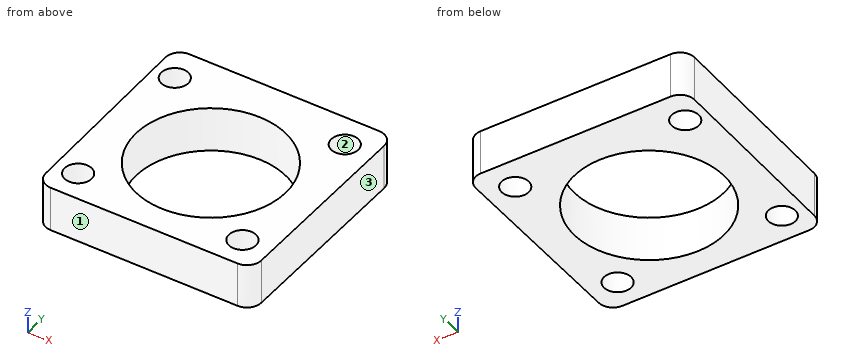
```python
from build123d import *

# Parameters (mm, degrees)
F0_R     = 7.5
F0_R_2   = 41.5
F1_DEPTH = 25


with BuildPart() as f1:
    # F0 (on Top) → F1 (new body)
    with BuildSketch(Plane.XY):
        with BuildLine():
            ThreePointArc((-59.925168, -48.84305), (-57.53589, -54.413699), (-51.926274, -56.709997))
            Line((-51.926274, -56.709997), (52.20569, -56.709997))
            ThreePointArc((52.20569, -56.709997), (57.862545, -54.366851), (60.20569, -48.709997))
            Line((60.20569, -48.709997), (60.20569, 55.273405))
            ThreePointArc((60.20569, 55.273405), (57.862545, 60.93026), (52.20569, 63.273405))
            Line((52.20569, 63.273405), (-53.655924, 63.273405))
            ThreePointArc((-53.655924, 63.273405), (-59.359626, 60.883021), (-61.654818, 55.140352))
            Line((-61.654818, 55.140352), (-59.925168, -48.84305))
        make_face()
        with Locations((-47.246009, -40.616337)):
            Circle(F0_R, mode=Mode.SUBTRACT)
        with Locations((44.347703, -40.616337)):
            Circle(F0_R, mode=Mode.SUBTRACT)
        Circle(F0_R_2, mode=Mode.SUBTRACT)
        with Locations((-49.459223, 44.541564)):
            Circle(F0_R, mode=Mode.SUBTRACT)
        with Locations((44.347703, 45.987621)):
            Circle(F0_R, mode=Mode.SUBTRACT)
    extrude(amount=-F1_DEPTH)


solid = f1.part
```
CAD build for the part. Positions are in the model's coordinates, mm. Face numbers are marked on the shaded views. Coordinates: 2 decimals unless noted, no trailing zeros. Order: outer loops, then holes, each group sorted by start corner. A loop starts at its lowest first (then second) coordinate and runs counter-clockwise, first axis right, second up. Notation, with made-up numbers: (69, 23) -> (113, 23) arc R8 ccw to (113, 34) -> close; hole circle Ø10 at (53, 8.5). An arc over 180 degrees is marked (long way). Use one line per item in the form item = value. Start each with the question number.
1) Band-saw the part on B-B on y = 0. Give the cut face in (x, z).
2) Band-saw the part on A-A on x = 0. Give the cut face in (y, z).
3) Drill centre lines: L1, parallel to Y at x = 0, z = -15.5; L2, parallel to Y at x = 46, z = -6; L3, parallel to X at y = 44, z = -12.25. Where is each one in solid material? Low to high. Write a range as [from, to].
4) Drop flat-ended pins along their axis: pin 1 (1.5 mm diameter, centred on y = 37, z = -7, fed in from -X); pin 2 (5 mm diameter, centred on y = -8.5, z = -15.5, fed in from -X); pin 3 (1 mm diameter, centred on y = 9.5, z = -8.5, fed in from -X). Give the stop position or say it passes through.
5) Pull direction X, two halves, no side cores. Call the marked faces 1, 2 and 3: +X half, -X half, draft (parallel to the pull), parting line (faces both ways), or undercut.
6) Band-saw the part on C-C on y = -43. Give the cut face in (x, z), then the cut area to 3 significant figures.
7) Band-saw the part on D-D on x = -48. Give the cut face in (y, z), then the cut area to 3 significant figures.
Entries:
q1.outline = (-60.74, -25) -> (-41.5, -25) -> (-41.5, 0) -> (-60.74, 0) -> close; (41.5, -25) -> (60.21, -25) -> (60.21, 0) -> (41.5, 0) -> close
q2.outline = (-56.71, -25) -> (-41.5, -25) -> (-41.5, 0) -> (-56.71, 0) -> close; (41.5, -25) -> (63.27, -25) -> (63.27, 0) -> (41.5, 0) -> close
q3.L1 = [-56.71, -41.5], [41.5, 63.27]
q3.L2 = [-56.71, -47.93], [-33.3, 38.67], [53.3, 63.27]
q3.L3 = [-61.47, -56.94], [-41.98, 37.12], [51.58, 60.21]
q4.pin_1 = -61.37
q4.pin_2 = -60.64
q4.pin_3 = -60.9
q5.face_1 = draft
q5.face_2 = undercut
q5.face_3 = +X half
q6.outline = (-60.02, -25) -> (-54.36, -25) -> (-54.36, 0) -> (-60.02, 0) -> close; (-40.13, -25) -> (37.24, -25) -> (37.24, 0) -> (-40.13, 0) -> close; (51.46, -25) -> (60.21, -25) -> (60.21, 0) -> (51.46, 0) -> close
q6.area = 2,290 mm2
q7.outline = (-56.71, -25) -> (-48.08, -25) -> (-48.08, 0) -> (-56.71, 0) -> close; (-33.15, -25) -> (37.18, -25) -> (37.18, 0) -> (-33.15, 0) -> close; (51.9, -25) -> (63.27, -25) -> (63.27, 0) -> (51.9, 0) -> close
q7.area = 2,260 mm2
